Geometry: final body of the model. Coordinates: model frame, mm. A direction names the side the tool comes from. Round coordinates to 2 decimals unless told otherwise and drop trailing zeros. Order: outer loops, then holes, each group sorted by start corner. A loop starts at its lowest first (then second) coordinate and runs counter-clockwise, first axis right, second up. Notation, with made-up numbers: M 37.25,-11.5 L 52.25,-11.5 A34 ccw 52.25,19.5 Z; hole C 14,-20.75 d5. An arc over 180 degrees is marked long. Put each result on its own line as item: value. Start each with the question number.
1) Section A-A, the plane x = 1.05. Return loops of the section in (y, z).
2) Section C-C, the plane y = 8. Return loops of the section in (x, z) (3 decimals).
3) Draft query along Y for faces 1 (the flat face through (2, -10, -12)), 2 (the cylindrical face through (1.6, -5.5, -0.1)), 3 (the cylindrical face through (1.57, 56.34, -24.61)), 4 (the flat face through (2, 44, 10)). Return one class per face: pulls with the +Y half, pulls with the -Y half, needs draft (parallel to the pull), parting line crosses it, or undercut.
4) Access query for faces 5 (the cylindrical face through (1.57, 96.99, 7.15)), 6 (the flat face through (2, 44, 5.5)). Directions: +Z, -Z, +X, -X, +Y, -Y. A direction counts if a zero-diameter tool reaches every point of the face in a straight line with its end or side. Return the directions, or none.
5) Material intervals for probe 1 along Z at (x, y) = (1.85, 55); probe 2 along Z at (x, y) = (1.05, 46); probe 3 along Z at (x, y) = (0.7, 53), sorted ascending. Write a range as [from, to].
6) Section D-D, the plane z = -22.5. Return loops of the section in (x, y) (3 decimals).
7) Section B-B, the plane y = 55. Return loops of the section in (x, z) (3 decimals), then the cut area to 3 significant figures.
Autodesk Fusion 360 part; units mm, degrees
sketch "Sketch1" plane through (0, 0, 0) normal (1, 0, 0) x (0, 1, 0)
  line L0 (-10, 0) -> (-10, -35)
  line L1 (-10, -35) -> (100, -35)
  line L2 (100, -35) -> (100, 0)
  line L3 (0, 10) -> (90, 10)
  line L4 (0, 5.5) -> (90, 5.5)
  line L5 (90, -5.5) -> (0, -5.5)
  arc A0 (0, 10) -> (-10, 0) centre (0, 0) ccw
  arc A1 (0, 5.5) -> (0, -5.5) centre (0, 0) ccw
  arc A2 (100, 0) -> (90, 10) centre (90, 0) ccw
  arc A3 (90, -5.5) -> (90, 5.5) centre (90, 0) ccw
  line L6 (-10, -35) -> (-10, -22.5) construction
  line L7 (-10, -22.5) -> (100, -22.5) construction
  line L8 (45, -22.5) -> (45, -35) construction
  circle A4 centre (15, -22.5) radius 2.5
  circle A5 centre (55, -22.5) radius 2.5
  dimension "d1" = 11
  dimension "d2" = 20
  dimension "d3" = 11
  dimension "d4" = 20
  dimension "d5" = 90
  dimension "d7" = 35
  dimension "d10" = 12.5
  dimension "d11" = 5
  dimension "d12" = 5
  dimension "d16" = 30
  dimension "d17" = 10
extrude "Extrude1" add sketch "Sketch1" along normal blind 3.175
fillet "Fillet1" radius 10 1 edges at (1.5875, -10, -35)
fillet "Fillet2" radius 30 1 edges at (1.5875, 100, -35)
Result sheet:
1. outline: M -10,-25 A10 ccw 0,-35 L 70,-35 A30 ccw 100,-5 L 100,0 A10 ccw 90,10 L 0,10 A10 ccw -10,0 Z; hole M 0,-5.5 L 90,-5.5 A5.5 ccw 90,5.5 L 0,5.5 A5.5 ccw Z; hole C 15,-22.5 d5; hole C 55,-22.5 d5
2. outline: M 0,-35 L 3.175,-35 L 3.175,-5.5 L 0,-5.5 Z; M 0,5.5 L 3.175,5.5 L 3.175,10 L 0,10 Z
3. face 1: pulls with the -Y half
3. face 2: undercut
3. face 3: undercut
3. face 4: needs draft
4. face 5: +Z, +X, -X, +Y
4. face 6: +X, -X
5. probe 1: z = [-35, -25], [-20, -5.5], [5.5, 10]
5. probe 2: z = [-35, -5.5], [5.5, 10]
5. probe 3: z = [-35, -24], [-21, -5.5], [5.5, 10]
6. outline: M 0,-10 L 3.175,-10 L 3.175,12.5 L 0,12.5 Z; M 0,17.5 L 3.175,17.5 L 3.175,52.5 L 0,52.5 Z; M 0,57.5 L 3.175,57.5 L 3.175,94.367 L 0,94.367 Z
7. outline: M 0,-35 L 3.175,-35 L 3.175,-25 L 0,-25 Z; M 0,-20 L 3.175,-20 L 3.175,-5.5 L 0,-5.5 Z; M 0,5.5 L 3.175,5.5 L 3.175,10 L 0,10 Z
7. area: 92.1 mm2
